The figure shows three views and two pictorial views of one solid part (mm, origin at its lowest corner). Answer the questions. Round coordinates to 2 decimals unless told otherwise and drop trailing zeros. Order: outer loops, then holes, each group sorted by start corner. A loop starts at its lowest first (then second) coordinate and runs counter-clockwise, first axis right, second up. Notation, with made-up numbers: (85.5, -1) - (104.5, -1) arc R23 ccw to (104.5, 8) - close; hole circle Ø4 at (4, 58.5). An arc over 180 degrees is marked (long way). Answer in a Markdown table with one row per item.
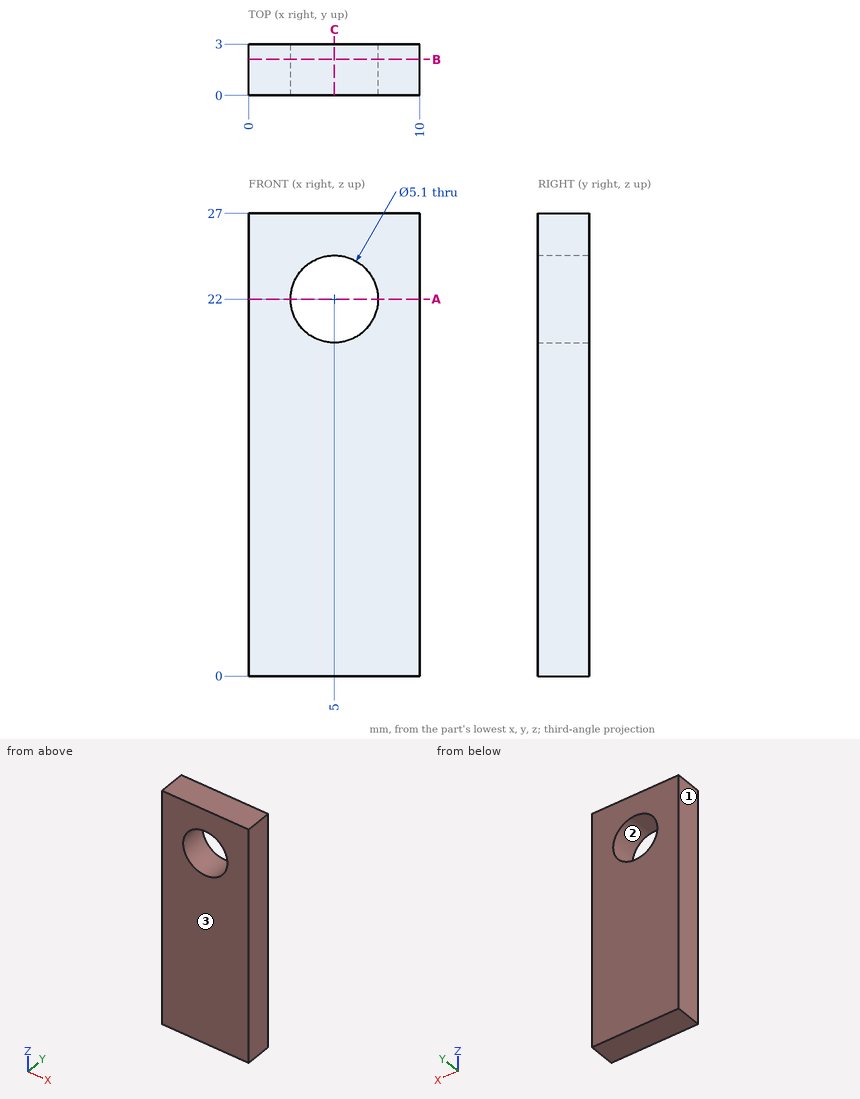
1) Find section C-C, the plane x = 5. Give the vertices of the cut face in (y, z).
Filled in:
| item | result |
|---|---|
| outline | (0, 0) - (3, 0) - (3, 19.45) - (0, 19.45) - close; (0, 24.55) - (3, 24.55) - (3, 27) - (0, 27) - close |
2) The mould has two halves that part along X. Classify the marked faces 1, 2 and 3: released by +X, released by -X, zero draft, split by the parting line, or undercut.
Filled in:
| item | result |
|---|---|
| face 1 | released by -X |
| face 2 | undercut |
| face 3 | zero draft |
3) Find the intervals of material crossed by probe 1 along Z at (x, y) = (5, 2.45); probe 2 along X at (y, z) = (2.15, 22); probe 3 along Z at (x, y) = (4.25, 1.15), in increasing order. Write a range as from..to.
Filled in:
| item | result |
|---|---|
| probe 1 | z = 0..19.45, 24.55..27 |
| probe 2 | x = 0..2.45, 7.55..10 |
| probe 3 | z = 0..19.56, 24.44..27 |
4) Find section A-A, the plane z = 22. Give the vertices of the cut face in (x, y).
Filled in:
| item | result |
|---|---|
| outline | (0, 0) - (2.45, 0) - (2.45, 3) - (0, 3) - close; (7.55, 0) - (10, 0) - (10, 3) - (7.55, 3) - close |
5) Find section B-B, the plane y = 2.1. Give the vertices of the cut face in (x, z).
Filled in:
| item | result |
|---|---|
| outline | (0, 0) - (10, 0) - (10, 27) - (0, 27) - close; hole circle Ø5.1 at (5, 22) |
